Verification items for the finished model (mm, model axes). Face numbers are marked on the shaded views. A direction names the side the tool comes from. Give positions to 0.01 mm unless a question says otherwise; leave off trailing zeros. Order: outer loops, then holes, each group sorted by start corner. A loop starts at its lowest first (then second) coordinate and runs counter-clockwise, first axis right, second up.
(1) Sectioned sample at C-C on z = -82.5. Record the cut outline in (x, y).
(2) Access from +Z, -Z, +X, -X, +Y, -Y to the whole of each face (thin tool, end or side, straight path). Record for the marked faces 1, 2 and 3.
(3) Sectioned sample at D-D on x = 0. Count the separate pieces of the cut face and the enclosed holes in it, plus the area to 3 significant figures.
(4) Mould release check, pull along Z, two halves, no side actions. Record for the marked faces 4, 5 and 6: pulls with the +Z half, pulls with the -Z half, needs draft (parallel to the pull), parting line crosses it, or undercut.
(5) Sectioned sample at A-A on y = -22. Record the cut outline in (x, z), plus the area to 3 significant figures.
(6) Scan lines: L1, parallel to Y at x = 0, z = -3.3; L2, parallel to Y at x = -1, z = -28.5; L3, parallel to Z at x = 11, y = 20.5. Record each from-to range of solid material in increasing order.
(7) Gauge pin test, flat ends, axial feed: pin 1 (10 mm diameter, centred on x = -15.5, y = 9, fed in from -Z); pin 2 (12 mm diameter, centred on y = -12.5, z = -43, fed in from -X); pin 3 (3 mm diameter, centred on x = -20.5, y = -21.5, fed in from -Z); pin 4 (5 mm diameter, centred on x = 0, y = -22, fed in from +Z). Record the tip position at first contact, or that the pin passes through.
```python
from build123d import *

# Parameters (mm, degrees)
F2_SIZE  = 2
F3_SIZE  = 1
F4_R     = 6
F5_DEPTH = 5
F6_R     = 2.1
F7_DEPTH = 10


with BuildPart() as f1:
    # F0 (on Front) → F1 (revolve)
    with BuildSketch(Plane.XZ):
        Polygon((0, -106), (0, 0), (-15, 0), (-15, -23), (-27, -23), (-27, -31), (-16.5, -31), (-16.5, -55), (-8.5, -55), (-8.5, -91), (-6, -91), (-6, -106), align=None)
    revolve(axis=Axis((0, 0, -53), (0, 0, 1)))

    # F2
    f2_edges = [f1.edges().sort_by_distance(p)[0] for p in [
        (15, 0, 0),
        (16.5, 0, -55),
    ]]
    chamfer(f2_edges, length=F2_SIZE)

    # F3
    f3_edges = [f1.edges().sort_by_distance(p)[0] for p in [
        (6, 0, -106),
    ]]
    chamfer(f3_edges, length=F3_SIZE)

    # F4 (on face) → F5 (cut)
    with BuildSketch(Plane.XY):
        Circle(F4_R)
    extrude(amount=-F5_DEPTH, mode=Mode.SUBTRACT)

    # F6 (on face) → F7 (cut)
    with BuildSketch(Plane.XY.offset(-23)):
        with Locations((0, 22)):
            Circle(F6_R)
        with Locations((-19.0525588833, 11)):
            Circle(F6_R)
        with Locations((-19.0525588833, -11)):
            Circle(F6_R)
        with Locations((0, -22)):
            Circle(F6_R)
        with Locations((19.0525588833, -11)):
            Circle(F6_R)
        with Locations((19.0525588833, 11)):
            Circle(F6_R)
    extrude(amount=-F7_DEPTH, mode=Mode.SUBTRACT)


solid = f1.part
```
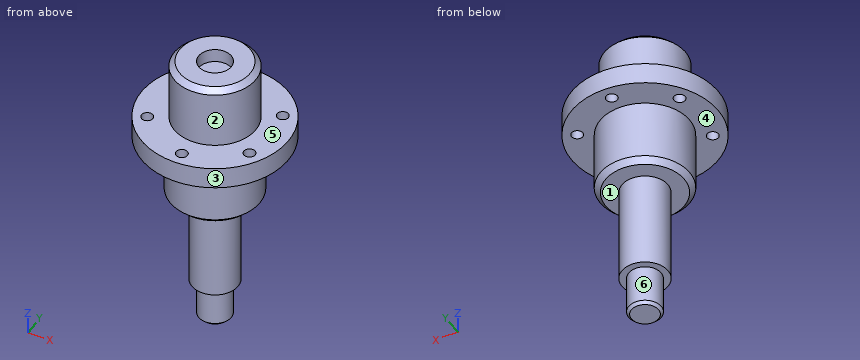
Ans:
1. outline: circle Ø17 at (0, 0)
2. face 1: -Z
2. face 2: +Z
2. face 3: +Z, -Z
3. separate pieces: 3
3. enclosed holes: 0
3. area: 2,570 mm2
4. face 4: pulls with the -Z half
4. face 5: pulls with the +Z half
4. face 6: needs draft
5. outline: (-15.65, -31) - (-2.1, -31) - (-2.1, -23) - (-15.65, -23) - close; (2.1, -31) - (15.65, -31) - (15.65, -23) - (2.1, -23) - close
5. area: 217 mm2
6. L1: y = -15 to -6, 6 to 15
6. L2: y = -26.98 to -23.85, -20.15 to 20.15, 23.85 to 26.98
6. L3: z = -31 to -23
7. pin 1: stops at z = -55
7. pin 2: stops at x = -15.17
7. pin 3: passes through
7. pin 4: stops at z = -23
